```python
from build123d import *

# Parameters (mm, degrees)
SKETCH1_R                      = 29.64
SKETCH1_R_2                    = 22.5
BOSS_EXTRUDE1_DEPTH            = 51
SKETCH1_4_W                    = 5.7
SKETCH1_4_H                    = 2.7
BOSS_EXTRUDE2_DEPTH            = 9.85
CIRPATTERN2_COUNT              = 3
BOSS_EXTRUDE3_DEPTH            = 3.175
CUT_EXTRUDE2_REACH             = 75.89
SKETCH7_R                      = 4.9125
CUT_EXTRUDE2_DIRECTION_2_DEPTH = 74.890335633
SKETCH8_W                      = 12.873355566
SKETCH8_H                      = 48.17275248
SKETCH8_R                      = 3.475
BOSS_EXTRUDE4_DEPTH            = 9
SKETCH1_3_W                    = 4.8
SKETCH1_3_H                    = 9.8
CUT_EXTRUDE1_DEPTH             = 23
CIRPATTERN1_COUNT              = 6
SKETCH11_W                     = 9
SKETCH11_H                     = 9
CUT_EXTRUDE21_DEPTH            = 29


with BuildPart() as part:
    # Sketch1 → Boss-Extrude1 (new body)
    with BuildSketch(Plane.XY):
        Circle(SKETCH1_R)
        Circle(SKETCH1_R_2, mode=Mode.SUBTRACT)
    extrude(amount=BOSS_EXTRUDE1_DEPTH)

    # Sketch1<4> → Boss-Extrude2 (add)
    with BuildSketch(Plane.XY):
        with Locations((0, 26.5)):
            Rectangle(SKETCH1_4_W, SKETCH1_4_H)
    boss_extrude2 = extrude(amount=-BOSS_EXTRUDE2_DEPTH)

    # CirPattern2: Boss-Extrude2 ×3 about axis
    cirpattern2_axis = Axis((0, 0, 0), (0, 0, 1))
    for i in range(1, CIRPATTERN2_COUNT):
        add(boss_extrude2.rotate(cirpattern2_axis, i * 360 / CIRPATTERN2_COUNT))

    # Sketch4 → Boss-Extrude3 (add)
    with BuildSketch(Plane.XY.offset(51)):
        Polygon((-6.436677783, -24.214121516), (6.436677783, -24.214121516), (6.436677783, -6.436677783), (24.214121516, -6.436677783), (24.214121516, 6.436677783), (6.436677783, 6.436677783), (6.436677783, 24.214121516), (-6.436677783, 24.214121516), (-6.436677783, 6.436677783), (-24.214121516, 6.436677783), (-24.214121516, -6.436677783), (-6.436677783, -6.436677783), align=None)
    extrude(amount=-BOSS_EXTRUDE3_DEPTH)

    # Sketch7 → Cut-Extrude2 (cut, up to next)
    with BuildSketch(Plane.XY.offset(51), mode=Mode.PRIVATE) as cut_extrude2_sk1:
        with Locations(Location((0, 0, 0), (0, 0, 180))):
            Circle(SKETCH7_R)
    cut_extrude2_tool1 = extrude(cut_extrude2_sk1.sketch, amount=-CUT_EXTRUDE2_REACH, mode=Mode.PRIVATE) & part.part
    add(cut_extrude2_tool1.solids().sort_by_distance((0, 0, 51))[0], mode=Mode.SUBTRACT)

    # Sketch7 → Cut-Extrude2 direction 2 (cut)
    with BuildSketch(Plane.XY.offset(51)):
        with Locations(Location((0, 0, 0), (0, 0, 180))):
            Circle(SKETCH7_R)
    extrude(amount=CUT_EXTRUDE2_DIRECTION_2_DEPTH, mode=Mode.SUBTRACT)

    # Sketch8 → Boss-Extrude4 (add)
    with BuildSketch(Plane.XY.offset(47.825)):
        Rectangle(SKETCH8_W, SKETCH8_H)
        Circle(SKETCH8_R, mode=Mode.SUBTRACT)
    extrude(amount=-BOSS_EXTRUDE4_DEPTH)

    # Sketch1<3> → Cut-Extrude1 (cut)
    with BuildSketch(Plane.XY):
        with Locations((25.9, 0)):
            Rectangle(SKETCH1_3_W, SKETCH1_3_H)
    cut_extrude1 = extrude(amount=CUT_EXTRUDE1_DEPTH, mode=Mode.SUBTRACT)

    # CirPattern1: Cut-Extrude1 ×6 about axis
    cirpattern1_axis = Axis((0, 0, 0), (0, 0, 1))
    for i in range(1, CIRPATTERN1_COUNT):
        add(cut_extrude1.rotate(cirpattern1_axis, i * 360 / CIRPATTERN1_COUNT), mode=Mode.SUBTRACT)

    # Sketch11 → Cut-Extrude21 (cut)
    with BuildSketch(Plane(origin=(0, 0, 51), x_dir=(-1, 0, 0), z_dir=(0, 0, -1))):
        with Locations((0, 10.0625)):
            Rectangle(SKETCH11_W, SKETCH11_H)
    cut_extrude21 = extrude(amount=CUT_EXTRUDE21_DEPTH, mode=Mode.SUBTRACT)

    # Mirror1: Cut-Extrude21 across plane
    add(cut_extrude21.mirror(Plane.ZX), mode=Mode.SUBTRACT)


solid = part.part
```
Check sheet for the modelled part. Datum: model origin and axes. Units: mm. A direction names the side the tool comes from. Round coordinates to 2 decimals unless told otherwise and drop trailing zeros. Order: outer loops, then holes, each group sorted by start corner. A loop starts at its lowest first (then second) coordinate and runs counter-clockwise, first axis right, second up.
1) Mould release check, pull along X, two halves, no side actions. Record for faces 6 (the flat face through (-13, 22, 23)), 7 (the flat face through (2.85, 26, -5)), 8 (the cylindrical face through (-6.425, -28.935, 25.143)): +X half, -X half, draft (parallel to the pull), parting line (faces both ways), or undercut.
2) Section check B-B (x = 0). Give the number of separate pieces and of enclosed holes in the cut face, and give its area (3 significant figures).
3) Go/stop test with flat-tipped pins: pin 1 Ø2.5 at (x, z) = (-10.5, 48.5) entering from +Y; pin 2 Ø5.5 at (x, z) = (-26, 9) entering from -Y; pin 3 Ø2 at (y, z) = (-18, 34.5) entering from -X; pin 4 Ø4 at (x, y) = (0, 0) entering from -Z (3 decimals). Record where each tip stops, or that it passes through.
4) Scan lines: line 1 (Y direction, x = 0, z = 42) (1 decimal); line 2 (Y direction, x = -15, z = 8); line 3 (Y direction, x = 0, z = 17). Record each from-to range of solid material in increasing order.
5) Section check A-A (y = 0). Record the boundary of the cut face in (x, z) (1 decimal).
6) Section check D-D (z = 20). Record the boundary of the cut face in (x, y).
7) Tool access check on faces 1 (the flat face through (28.3, 0, 11)), 2 (the flat face through (21.8, -12.54, -4.86)), 3 (the flat face through (-24.1, -13.96, -4.86)), 4 (the flat face through (23, -13, -9.85)), 5 (the flat face through (-4.5, 10, 45)). Record the directions out of +Z, -Z, +X, -X, +Y, -Y that give a thin tool (end or side, any length) a straight path to the whole face; none if there is none.
Result:
1. face 6: undercut
1. face 7: +X half
1. face 8: parting line
2. separate pieces: 4
2. enclosed holes: 0
2. area: 990 mm2
3. pin 1: stops at y = 28.16
3. pin 2: stops at y = -18.38
3. pin 3: stops at x = -24.28
3. pin 4: passes through
4. line 1: y = -29.6 to -14.6, -5.6 to -3.5, 3.5 to 5.6, 14.6 to 29.6
4. line 2: y = -25.56 to -24.02, -18.48 to -16.77, 16.77 to 18.48, 24.02 to 25.56
4. line 3: y = -29.64 to -22.5, 22.5 to 29.64
5. outline: (-29.6, 0) - (-28.3, 0) - (-28.3, 23) - (-23.5, 23) - (-23.5, 0) - (-22.5, 0) - (-22.5, 47.8) - (-6.4, 47.8) - (-6.4, 38.8) - (-3.5, 38.8) - (-3.5, 47.8) - (-4.9, 47.8) - (-4.9, 51) - (-29.6, 51) - close; (3.5, 38.8) - (6.4, 38.8) - (6.4, 47.8) - (22.5, 47.8) - (22.5, 0) - (23.5, 0) - (23.5, 23) - (28.3, 23) - (28.3, 0) - (29.6, 0) - (29.6, 51) - (4.9, 51) - (4.9, 47.8) - (3.5, 47.8) - close
6. outline: circle Ø59.28 at (0, 0); hole (-28.3, -4.9) - (-23.5, -4.9) - (-23.5, 4.9) - (-28.3, 4.9) - close; hole circle Ø45 at (0, 0); hole (-18.39, -22.06) - (-9.91, -26.96) - (-7.51, -22.8) - (-15.99, -17.9) - close; hole (-18.39, 22.06) - (-15.99, 17.9) - (-7.51, 22.8) - (-9.91, 26.96) - close; hole (7.51, -22.8) - (9.91, -26.96) - (18.39, -22.06) - (15.99, -17.9) - close; hole (7.51, 22.8) - (15.99, 17.9) - (18.39, 22.06) - (9.91, 26.96) - close; hole (23.5, -4.9) - (28.3, -4.9) - (28.3, 4.9) - (23.5, 4.9) - close
7. face 1: -Z
7. face 2: -Z, +Y
7. face 3: -Z, -X, -Y
7. face 4: -Z, +X, -X, +Y, -Y
7. face 5: +Z, -Z
